For this review, use the dimensioned drawing (mm, ordinates from the lowest corner) and the shaded views. A direction names the side the tool comes from. Coordinates: 2 decimals unless noted, no trailing zeros. Loops run counter-clockwise (first coordinate to the right, second up) from the corner with the lowest first, then second, coordinate; pieces in that order, holes last.
1. Take a section at D-D, the plane z = 4. State the section outline as (x, y) points.
2. Take a section at A-A, the plane z = 35. State the section outline as (x, y) points.
3. To check wall thickness, follow probe 1 along X at (y, z) = (6.5, 23.5); probe 2 along Y at (x, z) = (35, 25); probe 3 along Y at (x, z) = (15.5, 36.5). State the ranges of each line that lie inside material, in increasing order.
4. Take a section at B-B, the plane y = 17. State the section outline as (x, z) points.
5. Take a section at C-C, the plane x = 32. State the section outline as (y, z) points, then the cut area to 3 significant figures.
6. Clearance check with flat-ended pins moving along their axes: P1, Ø3, axis at x = 6, z = 15, coming from the -Y side; P2, Ø3, axis at y = 6, z = 25.5, coming from the +X side; P3, Ø8, axis at y = 4.5, z = 22.5, coming from the -X side; P4, Ø5, axis at x = 21, y = 28.5, coming from the -Z side. State where each tip first meets the part, or that it passes through.
7. Machinability: for the marked faces 1, 2, 3 and 4, which of the approach directions +Z, -Z, +X, -X, +Y, -Y give a long, thin tool a straight path to every point of the face, cutting with its end or side? Answer none if there is none.
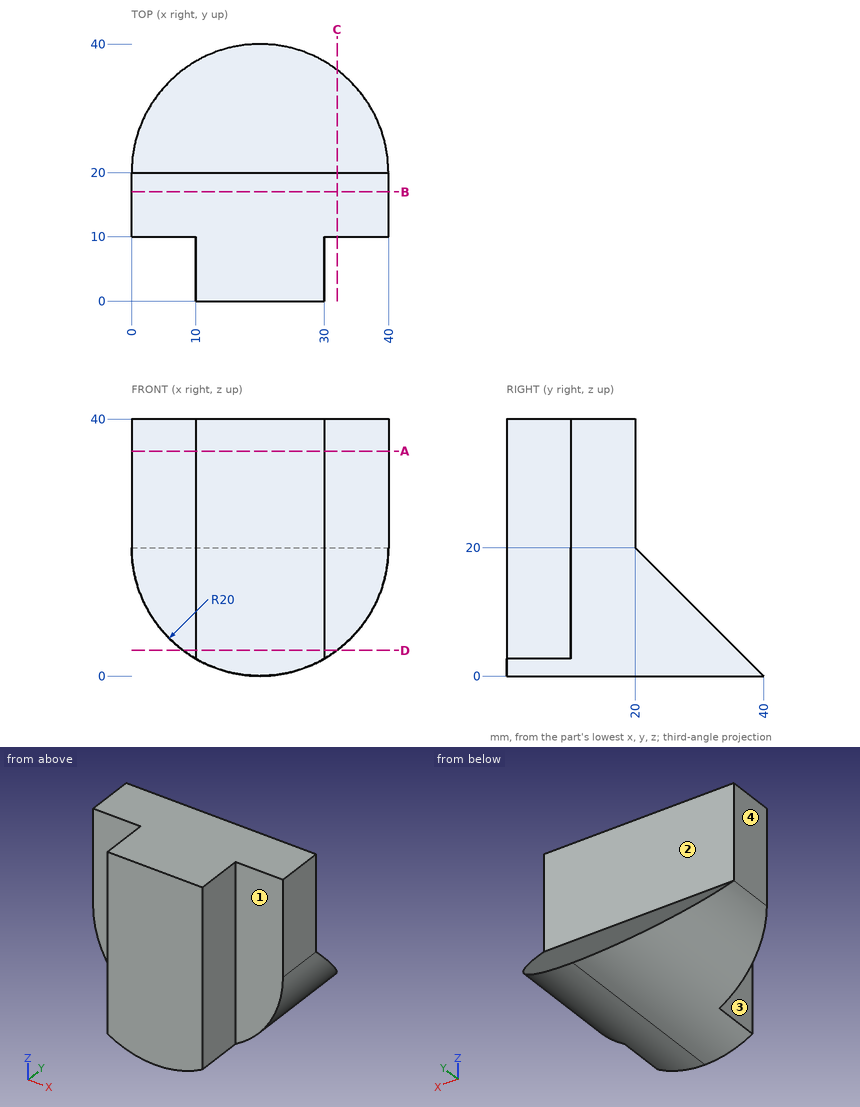
Results list:
1. outline: (8, 10) - (10, 10) - (10, 0) - (30, 0) - (30, 10) - (32, 10) - (32, 36) - (8, 36) - close
2. outline: (0, 10) - (10, 10) - (10, 0) - (30, 0) - (30, 10) - (40, 10) - (40, 20) - (0, 20) - close
3. probe 1: x = 10 to 30
3. probe 2: y = 10 to 20
3. probe 3: y = 0 to 20
4. outline: (0, 20) arc R20 ccw to (40, 20) - (40, 40) - (0, 40) - close
5. outline: (10, 4) - (36, 4) - (20, 20) - (20, 40) - (10, 40) - close
5. area: 488 mm2
6. P1: stops at y = 10
6. P2: stops at x = 30
6. P3: stops at x = 10
6. P4: stops at z = 0
7. face 1: +Z, -Z, +X, -Y
7. face 2: +Z, +X, -X, +Y
7. face 3: +Z, -Z, -X, -Y
7. face 4: +Z, -Z, -X, +Y, -Y
